The model under review builds one solid part; all positions refer to its coordinate system, in mm. Face numbers are marked on the shaded views. A direction names the side the tool comes from. Round coordinates to 2 decimals unless told otherwise and drop trailing zeros. Write each loop counter-clockwise with the first axis right and the second up, starting at its lowest first coordinate (ties: lowest second). Pieces come first, ordered by that corner, then holes. Notation, with made-up numbers: (-1.5, -25) - (53.5, -25) arc R24 ccw to (53.5, 12) - close; hole circle Ø6 at (30.5, -24.75). An arc over 180 degrees is marked (long way). Use one line per item in the form item = value.
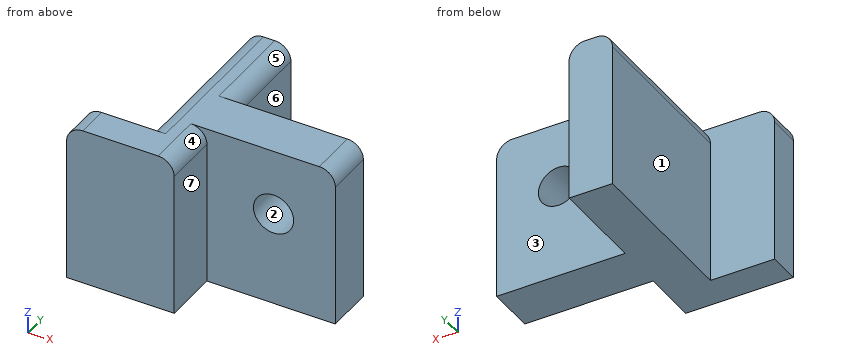
from build123d import *

# Parameters (mm, degrees)
AUFSATZ_LINEAR_AUSTRAGEN1_DEPTH      = 10
F_2_5_2_5_DURCHMESSER_BOHRUNG1_D     = 2.5
F_2_5_2_5_DURCHMESSER_BOHRUNG1_DEPTH = 5
F_2_5_2_5_DURCHMESSER_BOHRUNG1_TIP   = 0.751075774
VERRUNDUNG1_R                        = 1
VERRUNDUNG2_R                        = 1


with BuildPart() as part:
    # Skizze1 → Aufsatz-Linear austragen1 (new body)
    with BuildSketch(Plane.XY):
        Polygon((-2.7, 6), (0, 6), (0, 0), (8, 0), (8, -3), (0, -3), (0, -6.5), (-6.7, -6.5), (-6.7, -4.5), (-2.7, -4.5), align=None)
    extrude(amount=AUFSATZ_LINEAR_AUSTRAGEN1_DEPTH)

    # Ø2.5 (2.5) Durchmesser Bohrung1
    with Locations(Plane(origin=(0, -3, 0), x_dir=(-1, 0, 0), z_dir=(0, -1, 0))):
        with Locations((-4.15, -5.879543152)):
            Hole(F_2_5_2_5_DURCHMESSER_BOHRUNG1_D / 2, depth=F_2_5_2_5_DURCHMESSER_BOHRUNG1_DEPTH)
            with Locations((0, 0, -(F_2_5_2_5_DURCHMESSER_BOHRUNG1_DEPTH + F_2_5_2_5_DURCHMESSER_BOHRUNG1_TIP / 2))):  # 118° drill point
                Cone(0, F_2_5_2_5_DURCHMESSER_BOHRUNG1_D / 2, F_2_5_2_5_DURCHMESSER_BOHRUNG1_TIP, mode=Mode.SUBTRACT)

    # Verrundung1
    verrundung1_edges = [part.edges().sort_by_distance(p)[0] for p in [
        (-6.7, -5.5, 10),
        (0, -4.75, 10),
        (8, -1.5, 10),
        (0, 3, 10),
    ]]
    fillet(verrundung1_edges, radius=VERRUNDUNG1_R)

    # Verrundung2
    verrundung2_edges = [part.edges().sort_by_distance(p)[0] for p in [
        (-2.7, 0.75, 10),
    ]]
    fillet(verrundung2_edges, radius=VERRUNDUNG2_R)


solid = part.part
(1) Insertion check: P1, Ø1.5, axis at x = -4.5, z = 2.5, coming from the +Y side; P2, Ø1, axis at x = 3, z = 5, coming from the -Y side; P3, Ø2.5, axis at x = 2.5, z = 7, coming from the +Y side. Each pin has a flat end and moves straight along its axis. Give the tip position at first contact, or say it passes through.
Geometry results:
P1 = -4.5
P2 = -3
P3 = 0
(2) Add section A-A on x = 4.15. Write out the cut boundary in (y, z), then the cut area to 3 significant figures.
Geometry results:
outline = (-3, 0) - (0, 0) - (0, 4.63) - (-3, 4.63) - close; (-3, 7.13) - (0, 7.13) - (0, 10) - (-3, 10) - close
area = 22.5 mm2
(3) Add section D-D on z = 9.25. Write out the cut boundary in (x, y).
Geometry results:
outline = (-6.67, -6.5) - (-0.03, -6.5) - (-0.03, -3) - (7.97, -3) - (7.97, 0) - (-0.03, 0) - (-0.03, 6) - (-2.67, 6) - (-2.67, -4.5) - (-6.67, -4.5) - close
(4) The part is to be moulded in two halves that separate along X. For the marked faces 1, 2 and 3, say which applies: +X half, -X half, draft (parallel to the pull), parting line (faces both ways), or undercut.
Geometry results:
face_1 = -X half
face_2 = undercut
face_3 = draft
(5) Add section B-B on z = 5.5. Write out the cut boundary in (x, y), then the cut area to 3 significant figures.
Geometry results:
outline = (-6.7, -6.5) - (0, -6.5) - (0, -3) - (2.96, -3) - (2.96, 0) - (0, 0) - (0, 6) - (-2.7, 6) - (-2.7, -4.5) - (-6.7, -4.5) - close; (5.34, -3) - (8, -3) - (8, 0) - (5.34, 0) - close
area = 58.6 mm2
(6) Machinability: for the marked faces 4, 5, 6 and 7, which of the approach directions +Z, -Z, +X, -X, +Y, -Y give a long, thin tool a straight path to every point of the face, cutting with its end or side? Answer none if there is none.
Geometry results:
face_4 = +Z, +X, -Y
face_5 = +Z, +X, +Y
face_6 = +Z, -Z, +X, +Y
face_7 = +Z, -Z, +X, -Y
(7) To check wall thickness, follow L1, parallel to Y at x = 4.5, z = 7.5; L2, parallel to Z at x = 4.15, y = -1; L3, parallel to X at y = -2.5, z = 8.75. State the ranges of each line that lie inside material, in increasing order.
Geometry results:
L1 = -3 to 0
L2 = 0 to 4.63, 7.13 to 10
L3 = -2.7 to 8
(8) Add section C-C on y = -5.5. Write out the cut boundary in (x, z).
Geometry results:
outline = (-6.7, 0) - (0, 0) - (0, 9) arc R1 ccw to (-1, 10) - (-5.7, 10) arc R1 ccw to (-6.7, 9) - close
